from build123d import *


with BuildPart() as part:
    # Sketch2 → Revolve15 (revolve)
    with BuildSketch(Plane.XY):
        with BuildLine():
            ThreePointArc((-11.057536139, 6.861664444), (-8.978939648, 7.301650711), (-7.020479446, 6.477888049))
            ThreePointArc((-7.020479446, 6.477888049), (-3.561535652, 5.127833284), (0, 6.177787489))
            Line((0, 6.177787489), (0, -7.137400499))
            Line((0, -7.137400499), (-45.237397251, -7.137400499))
            Line((-45.237397251, -7.137400499), (-45.237397251, -4.99e-07))
            ThreePointArc((-45.237397251, -4.99e-07), (-34.450523736, 12.334918038), (-20.787740284, 3.288636819))
            ThreePointArc((-20.787740284, 3.288636819), (-17.488645172, 0.175380579), (-13.722322326, 2.703463882))
            ThreePointArc((-13.722322326, 2.703463882), (-12.908547636, 5.114921185), (-11.057536139, 6.861664444))
        make_face()
    revolve(axis=Axis((0.228383109, -0.616910329, 0), (0, 1, 0)))


solid = part.part
Verification items for the finished model (mm, model axes). Round coordinates to 2 decimals unless told otherwise and drop trailing zeros. Loops run counter-clockwise (first coordinate to the right, second up) from the corner with the lowest first, then second, coordinate; pieces in that order, holes last. Notation, with made-up numbers: (79, 85) - (131, 85) arc R22 cw to (131, 102) - close; hole circle Ø4 at (75, -35). An arc over 180 degrees is marked (long way). Use one line per item in the form item = value.
1. Section check B-B on y = 11. Record the cut outline in (x, z), and give its area (3 significant figures).
A:
outline = circle Ø77.68 at (0.23, 0); hole circle Ø54.39 at (0.23, 0)
area = 2,420 mm²
2. Section check A-A on y = -3. Record the cut outline in (x, z).
A:
outline = circle Ø90.93 at (0.23, 0); hole circle Ø0.46 at (0.23, 0)
3. Scan lines: probe 1 along Z at (x, y) = (1, 3.75); probe 2 along Z at (x, y) = (-3.5, 2.5); probe 3 along Y at (x, z) = (-16.5, -7). Record each from-to range of solid material in increasing order.
A:
probe_1 = -44.88 to -21.14, -13.74 to 13.74, 21.14 to 44.88
probe_2 = -45.06 to -20.48, -13.52 to 13.52, 20.48 to 45.06
probe_3 = -7.14 to 0.23
4. Gauge pin test, flat ends, axial feed: pin 1 Ø6 at (x, z) = (-10.5, 35.5) entering from +Y; pin 2 Ø3 at (x, y) = (30.5, 3) entering from +Z; pin 3 Ø10 at (y, z) = (-1, 16) entering from +X. Record the tip position at first contact, or that the pin passes through.
A:
pin_1 = 12.4
pin_2 = 34.81
pin_3 = 44.34
